```python
from build123d import *

# Parameters (mm, degrees)
SKETCH3_W           = 112.775418125
SKETCH3_H           = 62.141556926
BOSS_EXTRUDE1_DEPTH = 100
SKETCH4_W           = 11.300404478
SKETCH4_H           = 9.134771786
CUT_EXTRUDE1_DEPTH  = 100
CHAMFER2_START      = 50
CHAMFER2_OUTLINE_W  = 7.071067812
CHAMFER2_OUTLINE_H  = 100
CHAMFER2_DEPTH      = 4.115229923
SKETCH5_R           = 10
CUT_EXTRUDE2_DEPTH  = 100


with BuildPart() as part:
    # Sketch3 → Boss-Extrude1 (new body)
    with BuildSketch(Plane(origin=(0, 0, 0), x_dir=(1, 0, 0), z_dir=(0, 1, 0))):
        with Locations((4.603078291, 0.095897464)):
            Rectangle(SKETCH3_W, SKETCH3_H)
    extrude(amount=BOSS_EXTRUDE1_DEPTH)

    # Sketch4 → Cut-Extrude1 (cut)
    with BuildSketch(Plane(origin=(0, 100, 0), x_dir=(1, 0, 0), z_dir=(0, 1, 0))):
        with Locations((55.340585114, -26.407495106)):
            Rectangle(SKETCH4_W, SKETCH4_H)
    extrude(amount=-CUT_EXTRUDE1_DEPTH, mode=Mode.SUBTRACT)

    # Chamfer2: read off the stored shape, not the designer's step
    # Chamfer2 outline → Chamfer2 (add)
    with BuildSketch(Plane(origin=(0, 0, 0), x_dir=(0.707106781186548, 0, -0.707106781186547), z_dir=(0.707106781186547, 0, 0.707106781186548)).offset(CHAMFER2_START)):
        with Locations((19.693117364, 50)):
            Rectangle(CHAMFER2_OUTLINE_W, CHAMFER2_OUTLINE_H)
    extrude(amount=CHAMFER2_DEPTH)

    # Sketch5 → Cut-Extrude2 (cut)
    with BuildSketch(Plane(origin=(0, 100, 0), x_dir=(1, 0, 0), z_dir=(0, 1, 0))):
        with Locations(Location((0, 0, 0), (0, 0, 270))):
            Circle(SKETCH5_R)
    extrude(amount=-CUT_EXTRUDE2_DEPTH, mode=Mode.SUBTRACT)


solid = part.part
```
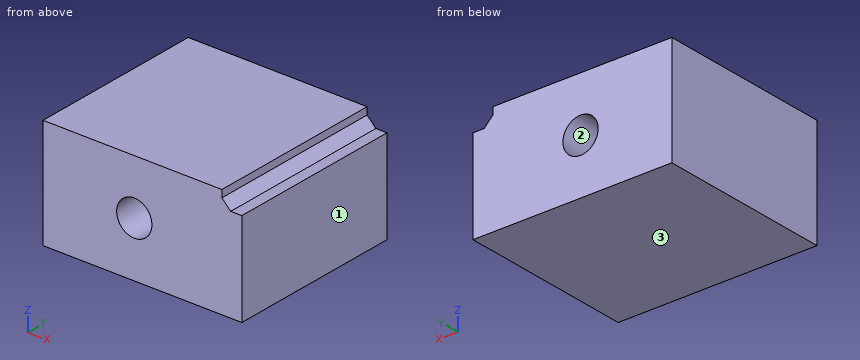
Check sheet for the modelled part. Datum: model origin and axes. Units: mm. Face numbers are marked on the shaded views. Round coordinates to 2 decimals unless told otherwise and drop trailing zeros. Loops run counter-clockwise (first coordinate to the right, second up) from the corner with the lowest first, then second, coordinate; pieces in that order, holes last. Notation, with made-up numbers: (78.5, 62) -> (108.5, 62) arc R26 ccw to (108.5, 79) -> close; hole circle Ø6 at (34.5, -4.5). An arc over 180 degrees is marked (long way). Answer in a Markdown table with one row per item.
Q1. Go/stop test with flat-tipped pins: P1, Ø8, axis at x = 47, z = -9, coming from the -Y side; P2, Ø3, axis at x = 57.5, y = 47, coming from the +Z side; P3, Ø3.5, axis at y = 32.5, z = 29, coming from the +X side. Record where each tip stops, or that it passes through.
Data:
| item | result |
|---|---|
| P1 | stops at y = 0 |
| P2 | stops at z = 21.84 |
| P3 | stops at x = 49.69 |
Q2. Sectioned sample at B-B on y = 42.5. Enter the section's corners in (x, z).
Data:
| item | result |
|---|---|
| outline | (-51.78, -31.17) -> (60.99, -31.17) -> (60.99, 21.84) -> (54.69, 21.84) -> (49.69, 26.84) -> (49.69, 30.97) -> (-51.78, 30.97) -> close; hole circle Ø20 at (0, 0) |
Q3. Release check for a two-part mould opening along Z. For the marked faces 1, 2 and 3 record: released by +Z, released by -Z, zero draft, split by the parting line, or undercut.
Data:
| item | result |
|---|---|
| face 1 | zero draft |
| face 2 | undercut |
| face 3 | released by -Z |
Q4. Sectioned sample at A-A on z = 0. Enter the section's corners in (x, y), then the cut area to 3 significant figures.
Data:
| item | result |
|---|---|
| outline | (-51.78, 0) -> (-10, 0) -> (-10, 100) -> (-51.78, 100) -> close; (10, 0) -> (60.99, 0) -> (60.99, 100) -> (10, 100) -> close |
| area | 9,280 mm^2 |
Q5. Thickness scan on L1, parallel to X at y = 62.5, z = 0; L2, parallel to X at y = 89.5, z = 28.5; L3, parallel to X at y = 71.5, z = -3. Record the ranges inside material, lowest first.
Data:
| item | result |
|---|---|
| L1 | x = -51.78 to -10, 10 to 60.99 |
| L2 | x = -51.78 to 49.69 |
| L3 | x = -51.78 to -9.54, 9.54 to 60.99 |
Q6. Sectioned sample at C-C on x = 0. Enter the section's corners in (y, z).
Data:
| item | result |
|---|---|
| outline | (0, -31.17) -> (100, -31.17) -> (100, -10) -> (0, -10) -> close; (0, 10) -> (100, 10) -> (100, 30.97) -> (0, 30.97) -> close |
